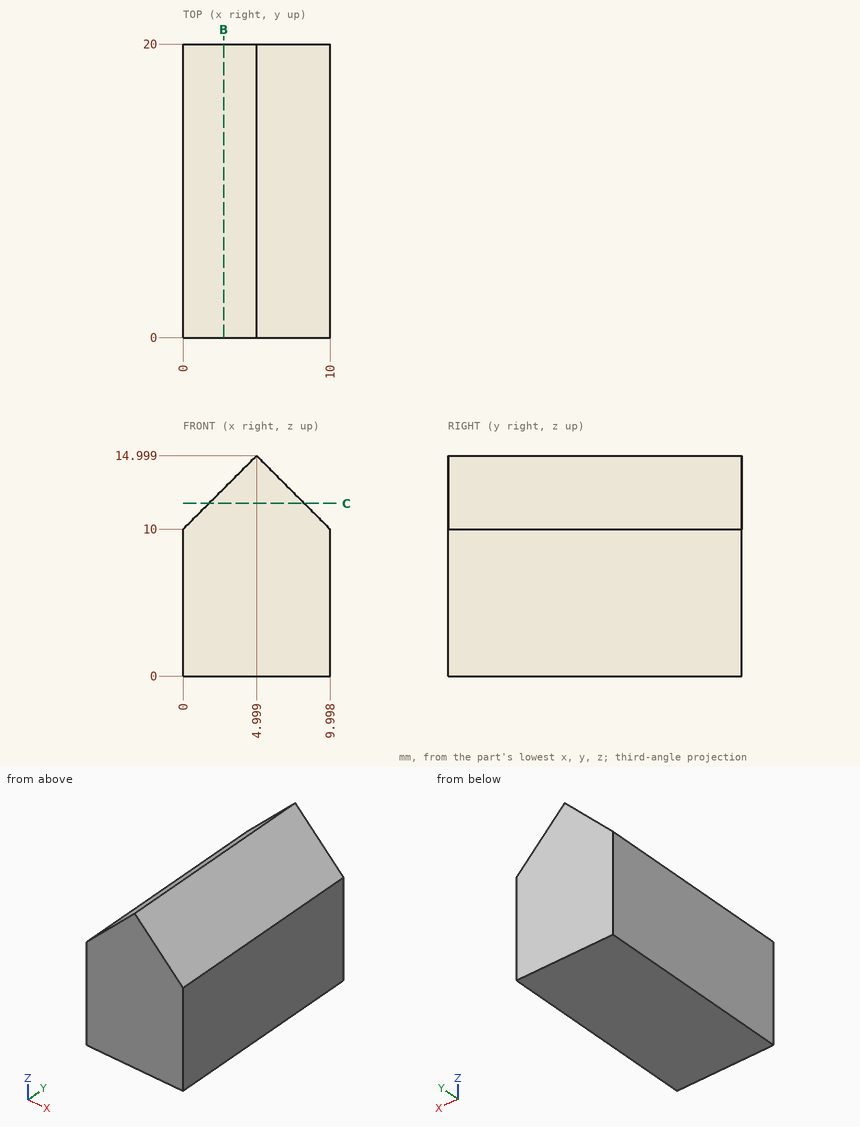
Drawing for the job (mm, zero at the part's lowest x, y, z). Give positions to 0.01 mm unless a question says otherwise; leave off trailing zeros. Write each loop counter-clockwise with the first axis right and the second up, starting at its lowest first coordinate (ties: lowest second). Pieces come first, ordered by that corner, then holes. Notation, with made-up numbers: (41.5, -13.5) - (72.5, -13.5) arc R31 ccw to (72.5, 25.5) - close; hole circle Ø6 at (4, 60). An arc over 180 degrees is marked (long way). Answer as CSV lines item,"result".
Q1. Band-saw the part on B-B (x = 2.75). Give the cut face in (y, z), and give its area (3 significant figures).
Result set:
outline,"(0, 0) - (20, 0) - (20, 12.75) - (0, 12.75) - close"
area,"255 mm²"
Q2. Band-saw the part on C-C (z = 11.75). Give the cut face in (x, y), and give its area (3 significant figures).
Result set:
outline,"(1.75, 0) - (8.25, 0) - (8.25, 20) - (1.75, 20) - close"
area,"130 mm²"
Q3. Drill centre lines: line 1 (X direction, y = 12.75, z = 13.75); line 2 (X direction, y = 15, z = 10.25); line 3 (Z direction, x = 8.5, y = 6.25). Where is each one in solid material? Low to high. Write a range as from..to.
Result set:
line 1,"3.75..6.25"
line 2,"0.25..9.75"
line 3,"0..11.5"
Q4. Flat gauge pins, fed straight in: pin 1 Ø4 at (x, z) = (5, 3.5) entering from -Y; pin 2 Ø2 at (y, z) = (8, 13.5) entering from +X. Where does each tip first touch, or does it go through?
Result set:
pin 1,"y = 0"
pin 2,"x = 7.5"
